CAD build for the part. Positions are in the model's coordinates, mm. A direction names the side the tool comes from. Give positions to 0.01 mm unless a question says otherwise; leave off trailing zeros. Loops run counter-clockwise (first coordinate to the right, second up) from the corner with the lowest first, then second, coordinate; pieces in that order, holes last. Notation, with made-up numbers: (75.25, 35) -> (79.25, 35) arc R6 cw to (79.25, 42) -> close; hole circle Ø7 at (1, -1). An arc over 180 degrees is marked (long way). Use one line per item in the form item = value.
```python
from build123d import *

# Parameters (mm, degrees)
EXTRUDE_1_DEPTH     = 4
SKETCH_2_R          = 4.5
EXTRUDE_2_DEPTH     = 1.9
SKETCH_3_R          = 3
CUT_EXTRUDE_1_DEPTH = 20
FILLET_1_R          = 1
FILLET_3_R          = 0.5


with BuildPart() as part:
    # 草图1 → 凸台-拉伸1 (new body)
    with BuildSketch(Plane(origin=(0, 0, 0), x_dir=(1, 0, 0), z_dir=(0, 1, 0))):
        Polygon((0, -5.773502692), (5, -2.886751346), (5, 2.886751346), (0, 5.773502692), (-5, 2.886751346), (-5, -2.886751346), align=None)
    extrude(amount=EXTRUDE_1_DEPTH)

    # 草图2 → 凸台-拉伸2 (add)
    with BuildSketch(Plane(origin=(0, 4, 0), x_dir=(1, 0, 0), z_dir=(0, 1, 0))):
        with Locations(Location((0, 0, 0), (0, 0, 90))):
            Circle(SKETCH_2_R)
    extrude(amount=EXTRUDE_2_DEPTH)

    # 草图3 → 切除-拉伸1 (cut)
    with BuildSketch(Plane(origin=(0, 5.9, 0), x_dir=(1, 0, 0), z_dir=(0, 1, 0))):
        with Locations(Location((0, 0, 0), (0, 0, 270))):
            Circle(SKETCH_3_R)
    extrude(amount=-CUT_EXTRUDE_1_DEPTH, mode=Mode.SUBTRACT)

    # 圆角1
    fillet_1_edges = [part.edges().sort_by_distance(p)[0] for p in [
        (0, 5.9, 4.5),
    ]]
    fillet(fillet_1_edges, radius=FILLET_1_R)

    # 圆角3
    fillet_3_edges = [part.edges().sort_by_distance(p)[0] for p in [
        (5, 4, 0),
        (2.5, 4, -4.330127019),
        (-2.5, 4, -4.330127019),
        (-5, 4, 0),
        (-2.5, 4, 4.330127019),
        (-5, 0, 0),
        (-2.5, 0, -4.330127019),
        (2.5, 0, -4.330127019),
        (5, 0, 0),
        (2.5, 0, 4.330127019),
        (-2.5, 0, 4.330127019),
        (2.5, 4, 4.330127019),
    ]]
    fillet(fillet_3_edges, radius=FILLET_3_R - 0.0001)  # a hair under: the kernel refuses the full size


solid = part.part
```
1. Drill centre lines: line 1 (X direction, y = 3.35, z = -1.5); line 2 (X direction, y = 4.85, z = -0.5); line 3 (Z direction, x = 1, y = 4.6). Where is each one in solid material? Low to high.
Result sheet:
line_1 = -5 to -2.6, 2.6 to 5
line_2 = -4.47 to -2.96, 2.96 to 4.47
line_3 = -4.39 to -2.83, 2.83 to 4.39
2. Drop flat-ended pins along their axis: P1, Ø5.5, axis at x = 0, z = 0, coming from the +Y side; P2, Ø5, axis at x = -0.5, z = 0.5, coming from the +Y side. Give the stop position or say it passes through.
Result sheet:
P1 = through
P2 = 5.9
3. Mould opens along Z. For faces 3 (the cylindrical face through (0.9, 2.99, 2.86)), 4 (the cylindrical face through (-2.46, 3.857, -4.18)), 5 (the cylindrical face through (-2.39, 3.86, 4.22)) say: pulls with the +Z half, pulls with the -Z half, needs draft (parallel to the pull), parting line crosses it, or undercut.
Result sheet:
face_3 = undercut
face_4 = pulls with the -Z half
face_5 = pulls with the +Z half
4. Cut at A-A, the plane y = 1.2. Write the cut outline in (x, z), then the cut area to 3 significant figures.
Result sheet:
outline = (-5, -2.89) -> (0, -5.77) -> (5, -2.89) -> (5, 2.89) -> (0, 5.77) -> (-5, 2.89) -> close; hole circle Ø6 at (0, 0)
area = 58.3 mm^2
5. Tool access for faces 1 (the cylindrical face through (-1.352, 4.444, -4.292)), 2 (the cylindrical face through (-2.46, 0.15, -4.19)): list every direction of +Z, -Z, +X, -X, +Y, -Y with a clear straight run to the whole face (end or side of a thin tool).
Result sheet:
face_1 = +Y
face_2 = -Z, -X, -Y
